```python
from build123d import *

# Parameters (mm, degrees)
CROQUIS1_R              = 1.25
SALIENTE_EXTRUIR1_DEPTH = 1
CROQUIS2_W              = 1
CROQUIS2_H              = 6
SALIENTE_EXTRUIR2_DEPTH = 6
REDONDEO1_RADIUS        = 3
REDONDEO1_LENGTH        = 1
CORTAR_EXTRUIR1_REACH   = 12.689
CROQUIS3_R              = 1.25
REDONDEO2_R             = 1.5


with BuildPart() as part:
    # Croquis1 → Saliente-Extruir1 (new body)
    with BuildSketch(Plane.XY):
        with BuildLine():
            Line((-5, -3), (5, -3))
            ThreePointArc((5, -3), (6.414213562, -2.414213562), (7, -1))
            Line((7, -1), (7, 1))
            ThreePointArc((7, 1), (6.414213562, 2.414213562), (5, 3))
            Line((5, 3), (-5, 3))
            ThreePointArc((-5, 3), (-6.414213562, 2.414213562), (-7, 1))
            Line((-7, 1), (-7, -1))
            ThreePointArc((-7, -1), (-6.414213562, -2.414213562), (-5, -3))
        make_face()
        with Locations((-5, 0)):
            Circle(CROQUIS1_R, mode=Mode.SUBTRACT)
        with Locations((5, 0)):
            Circle(CROQUIS1_R, mode=Mode.SUBTRACT)
    extrude(amount=SALIENTE_EXTRUIR1_DEPTH)

    # Croquis2 → Saliente-Extruir2 (add)
    with BuildSketch(Plane.XY.offset(1)):
        Rectangle(CROQUIS2_W, CROQUIS2_H)
    extrude(amount=SALIENTE_EXTRUIR2_DEPTH)

    # Redondeo1: full round fillet: the end face becomes a half cylinder, R = half its width
    redondeo1_face = Plane((0, 0, 7), x_dir=(-1, 0, 0), z_dir=(0, 0, 1))  # on the end face: x along it, z out of the body
    redondeo1_slab = redondeo1_face.offset(-REDONDEO1_RADIUS / 2) * Box(REDONDEO1_LENGTH, 2 * REDONDEO1_RADIUS, REDONDEO1_RADIUS, mode=Mode.PRIVATE)  # the body's end, R deep
    redondeo1_round = Plane((0, 0, 4), x_dir=(0, 0, 1), z_dir=(-1, 0, 0)) * Cylinder(REDONDEO1_RADIUS, REDONDEO1_LENGTH, mode=Mode.PRIVATE)  # its axis R under the face
    add(redondeo1_slab - redondeo1_round, mode=Mode.SUBTRACT)

    # Croquis3 → Cortar-Extruir1 (cut, up to next)
    with BuildSketch(Plane.ZY.offset(0.5), mode=Mode.PRIVATE) as cortar_extruir1_sk1:
        with Locations((3.75, 0)):
            Circle(CROQUIS3_R)
    cortar_extruir1_tool1 = extrude(cortar_extruir1_sk1.sketch, amount=-CORTAR_EXTRUIR1_REACH, mode=Mode.PRIVATE) & part.part
    add(cortar_extruir1_tool1.solids().sort_by_distance((-0.5, 0, 3.75))[0], mode=Mode.SUBTRACT)

    # Redondeo2
    redondeo2_edges = [part.edges().sort_by_distance(p)[0] for p in [
        (0.5, 0, 1),
        (-0.5, 0, 1),
    ]]
    fillet(redondeo2_edges, radius=REDONDEO2_R - 0.0001)  # a hair under: the kernel refuses the full size


solid = part.part
```
The listing builds one solid part. Answer for the finished solid, in the listing's coordinates (mm). A direction names the side the tool comes from. Give positions to 0.01 mm unless a question says otherwise; leave off trailing zeros. Write each loop counter-clockwise with the first axis right and the second up, starting at its lowest first coordinate (ties: lowest second). Pieces come first, ordered by that corner, then holes. Notation, with made-up numbers: (-10, 89) - (35, 89) arc R31 cw to (35, 114) - close; hole circle Ø2 at (-22, -14.75). An arc over 180 degrees is marked (long way). Use one line per item in the form item = value. Start each with the question number.
1) Find section D-D on x = 2.75. Determine the outline of the cut face in (y, z).
2) Find section C-C on y = 2.65. Determine the outline of the cut face in (x, z).
3) Find section B-B on y = 0. Count the separate pieces of the cut face and the enclosed holes in it, plus the area to 3 significant figures.
4) Consider line 1 along Y through (x, z) = (5, 0.6); line 2 along Z through (x, y) = (-5.5, 2.35); line 3 along X through (y, z) = (-1.45, 6). Determine where each line is inside the solid, lowest interval first. Write a range as from..to.
5) Find section A-A on z = 3.75. Determine the outline of the cut face in (x, y).
6) A tool of negligible diameter and unlimited length cuts with its end or side. For faces 5 (the face through (-7, 0, 0.5)), 6 (the face through (0.5, 0, 5.2)), 7 (the face through (-0.5, 0, 5.2)), from which of +Z, -Z, +X, -X, +Y, -Y can it reach the whole face along a straight path? Write none if from no direction.
7) The mould has two halves that part along Z. Classify faces 1 (the face through (0, 0, 5)), 2 (the face through (3.75, 0.05, 0.49)), 3 (the face through (0, 0, 7)), 4 (the face through (0, 0, 0)): pulls with the +Z half, pulls with the -Z half, needs draft (parallel to the pull), parting line crosses it, or undercut.
8) Flat-ended cylindrical pins translate along their axes: pin 1 Ø1 at (x, y) = (-3, 1) entering from +Z; pin 2 Ø1.4 at (y, z) = (-1, 6) entering from -X. Find the tip coordinate at first contact, or state that the pin passes through.
Geometry results:
q1.outline = (-3, 0) - (3, 0) - (3, 1) - (-3, 1) - close
q2.outline = (-6.13, 0) - (6.13, 0) - (6.13, 1) - (2, 1) arc R1.5 cw to (0.5, 2.5) - (0.5, 5.41) - (-0.5, 5.41) - (-0.5, 2.5) arc R1.5 cw to (-2, 1) - (-6.13, 1) - close
q3.separate_pieces = 4
q3.enclosed_holes = 0
q3.area = 13.5 mm2
q4.line_1 = -3..-1.25, 1.25..3
q4.line_2 = 0..1
q4.line_3 = -0.5..0.5
q5.outline = (-0.5, -3) - (0.5, -3) - (0.5, -1.25) - (-0.5, -1.25) - close; (-0.5, 1.25) - (0.5, 1.25) - (0.5, 3) - (-0.5, 3) - close
q6.face_5 = +Z, -Z, -X, +Y, -Y
q6.face_6 = +Z, +X, +Y, -Y
q6.face_7 = +Z, -X, +Y, -Y
q7.face_1 = undercut
q7.face_2 = needs draft
q7.face_3 = pulls with the +Z half
q7.face_4 = pulls with the -Z half
q8.pin_1 = 1
q8.pin_2 = -0.5
